from build123d import *

# Parameters (mm, degrees)
F0_W     = 6.35
F0_H     = 6.35
F1_DEPTH = 4.7625


with BuildPart() as f1:
    # F0 (on Front) → F1 (new body)
    with BuildSketch(Plane.XZ):
        Polygon((-33.332054, 31.175699), (-38.888304, 28.109566), (-38.888304, 21.759566), (-33.332054, 18.685385), (-27.775804, 21.759566), (-27.775804, 28.109566), align=None)
        with Locations((-33.332054, 24.934566)):
            Rectangle(F0_W, F0_H, mode=Mode.SUBTRACT)
    extrude(amount=F1_DEPTH)


solid = f1.part
The model under review builds one solid part; all positions refer to its coordinate system, in mm. A direction names the side the tool comes from. Round coordinates to 2 decimals unless told otherwise and drop trailing zeros. Loops run counter-clockwise (first coordinate to the right, second up) from the corner with the lowest first, then second, coordinate; pieces in that order, holes last. Notation, with made-up numbers: (26, 32.5) -> (47, 32.5) arc R19 ccw to (47, 37.5) -> close; hole circle Ø6 at (-31.5, 63.5). An arc over 180 degrees is marked (long way). Return JSON: item names as keys, results as strings.
(1) The part is to be moulded in two halves that separate along Z. For faces 3 (the flat face through (-33, -4.762, 21)), 4 (the flat face through (-36.149, -2.348, 20.244)), 5 (the flat face through (-33, -2, 21.76)), say which applies: released by +Z, released by -Z, zero draft, split by the parting line, or undercut.
Solved:
{"face 3": "zero draft", "face 4": "released by -Z", "face 5": "undercut"}
(2) Add section B-B on y = -1.35. Write out the cut boundary in (x, z), plus the area to 3 significant figures.
Solved:
{"outline": "(-38.89, 21.76) -> (-33.33, 18.69) -> (-27.78, 21.76) -> (-27.78, 28.11) -> (-33.33, 31.18) -> (-38.89, 28.11) -> close; hole (-36.51, 21.76) -> (-30.16, 21.76) -> (-30.16, 28.11) -> (-36.51, 28.11) -> close", "area": "64.4 mm2"}
(3) For faces 1 (the flat face through (-27.776, -2, 25)), 2 (the flat face through (-36.507, -2, 25)), list the 3-axis set-ups (+Z, -Z, +X, -X, +Y, -Y) from which the entire face can be reached by the end or side of a thin tool; tool diameter is ignored.
Solved:
{"face 1": "+Z, -Z, +X, +Y, -Y", "face 2": "+Y, -Y"}
(4) Add section A-A on z = 23.5. Write out the cut boundary in (x, y).
Solved:
{"outline": "(-38.89, -4.76) -> (-36.51, -4.76) -> (-36.51, 0) -> (-38.89, 0) -> close; (-30.16, -4.76) -> (-27.78, -4.76) -> (-27.78, 0) -> (-30.16, 0) -> close"}
(5) Add section D-D on x = -29.25. Write out the cut boundary in (y, z).
Solved:
{"outline": "(-4.76, 20.94) -> (0, 20.94) -> (0, 28.92) -> (-4.76, 28.92) -> close"}
(6) Add section C-C on x = -30.5. Write out the cut boundary in (y, z), plus the area to 3 significant figures.
Solved:
{"outline": "(-4.76, 20.25) -> (0, 20.25) -> (0, 21.76) -> (-4.76, 21.76) -> close; (-4.76, 28.11) -> (0, 28.11) -> (0, 29.61) -> (-4.76, 29.61) -> close", "area": "14.3 mm2"}
(7) For line 1 (X direction, y = -4.25, z = 26.75); line 2 (Z direction, x = -31.5, y = -3.85); line 3 (Z direction, x = -32.25, y = -4.45), list the stretches that pass through material, from the lowest coordinate up.
Solved:
{"line 1": "-38.89 to -36.51, -30.16 to -27.78", "line 2": "19.7 to 21.76, 28.11 to 30.16", "line 3": "19.28 to 21.76, 28.11 to 30.58"}
